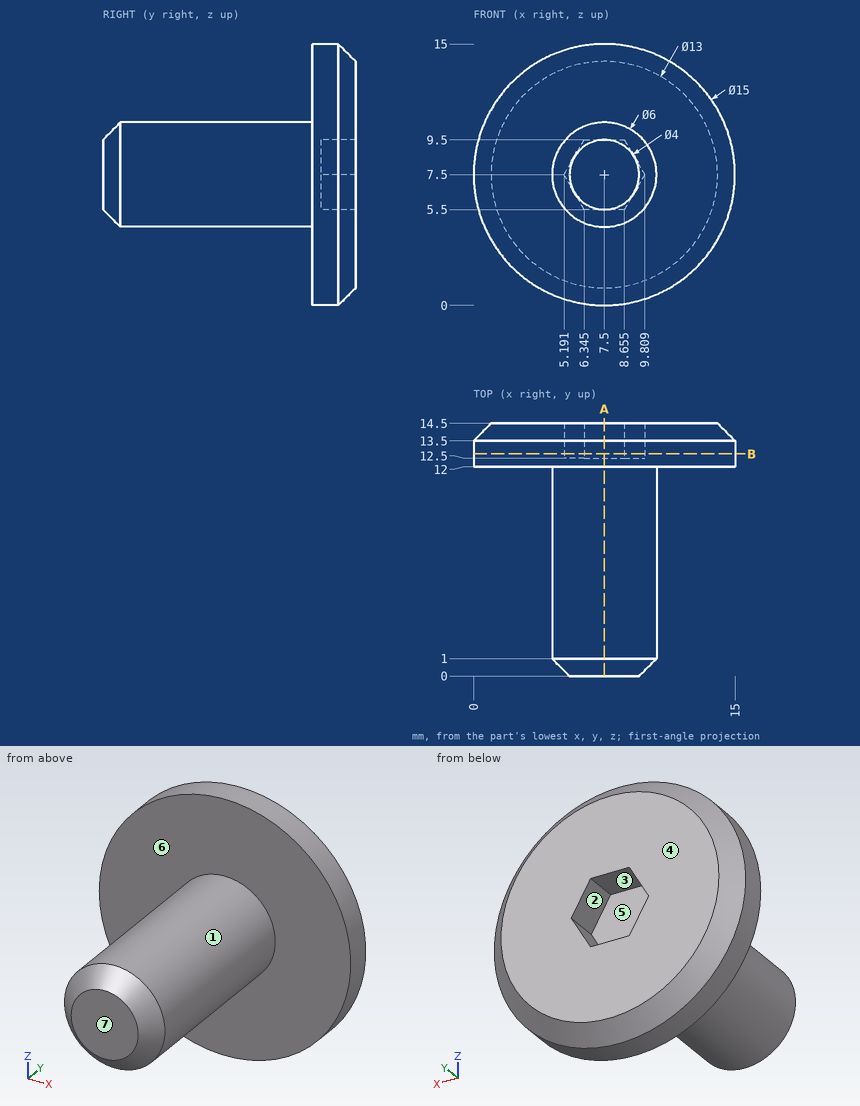
Verification items for this drawing (mm, ordinates from the low corner). A direction names the side the tool comes from. Give positions to 0.01 mm unless a question says otherwise; leave off trailing zeros. Write each loop counter-clockwise with the first axis right and the second up, starting at its lowest first coordinate (ties: lowest second). Pieces come first, ordered by that corner, then holes.
1) Material ranges on L1, parallel to Y at x = 12, z = 11; L2, parallel to Y at x = 6.75, z = 9; L3, parallel to X at y = 9.5, z = 7.5, recorded low to high.
2) Release check for a two-part mould opening along Z. For the marked faces 1, 2, 3 and 4 record: pulls with the +Z half, pulls with the -Z half, needs draft (parallel to the pull), parting line crosses it, or undercut.
3) Access from +Z, -Z, +X, -X, +Y, -Y to the whole of each face (thin tool, end or side, straight path). Record for the marked faces 5, 6 and 7.
4) Gauge pin test, flat ends, axial feed: pin 1 (4 mm diameter, centred on y = 9, z = 9.5, fed in from +X); pin 2 (5 mm diameter, centred on y = 4, z = 12, fed in from -X) (1 decimal); pin 3 (1.5 mm diameter, centred on y = 7.5, z = 10, fed in from -X). Record the tip position at first contact, or that the pin passes through.
5) Section check B-B, the plane y = 12.75. Record the boundary of the cut face in (x, z) (1 decimal), and give its area (3 significant figures).
6) Section check A-A, the plane x = 7.5. Record the boundary of the cut face in (y, z), and give its area (3 significant figures).
Computed:
1. L1: y = 12 to 14.5
1. L2: y = 0 to 12.5
1. L3: x = 4.5 to 10.5
2. face 1: parting line crosses it
2. face 2: undercut
2. face 3: undercut
2. face 4: needs draft
3. face 5: +Y
3. face 6: -Y
3. face 7: +Z, -Z, +X, -X, -Y
4. pin 1: stops at x = 10.5
4. pin 2: stops at x = 5.3
4. pin 3: stops at x = 5.06
5. outline: circle Ø15 at (7.5, 7.5); hole (5.2, 7.5) - (6.3, 5.5) - (8.7, 5.5) - (9.8, 7.5) - (8.7, 9.5) - (6.3, 9.5) - close
5. area: 163 mm2
6. outline: (0, 5.5) - (1, 4.5) - (12, 4.5) - (12, 0) - (13.5, 0) - (14.5, 1) - (14.5, 5.5) - (12.5, 5.5) - (12.5, 9.5) - (14.5, 9.5) - (14.5, 14) - (13.5, 15) - (12, 15) - (12, 10.5) - (1, 10.5) - (0, 9.5) - close
6. area: 99.5 mm2
